```python
from build123d import *

# Parameters (mm, degrees)
AUFSATZ_LINEAR_AUSTRAGEN2_DEPTH = 5
SCHNITT_LINEAR_AUSTRAGEN2_DEPTH = 38.080992435


with BuildPart() as part:
    # Skizze1 → Aufsatz-Linear austragen2 (new body)
    with BuildSketch(Plane.XY):
        with BuildLine():
            Line((0, 0), (0, 30))
            ThreePointArc((0, 30), (11.480502971, 27.716385975), (21.213203436, 21.213203436))
            Line((21.213203436, 21.213203436), (0, 0))
        make_face()
    extrude(amount=AUFSATZ_LINEAR_AUSTRAGEN2_DEPTH)

    # Skizze2 → Schnitt-Linear austragen2 (cut, through all)
    with BuildSketch(Plane.XY.offset(5)):
        with BuildLine():
            Line((14.142135624, 14.142135624), (21.213203436, 21.213203436))
            ThreePointArc((21.213203436, 21.213203436), (15, 25.980762114), (7.764571353, 28.977774789))
            Line((7.764571353, 28.977774789), (5.176380902, 19.318516526))
            ThreePointArc((5.176380902, 19.318516526), (10, 17.320508076), (14.142135624, 14.142135624))
        make_face()
    extrude(amount=-SCHNITT_LINEAR_AUSTRAGEN2_DEPTH, mode=Mode.SUBTRACT)


solid = part.part
```
Model file for the job. Use its own axes, mm. A direction names the side the tool comes from. Coordinates: 2 decimals unless noted, no trailing zeros. Order: outer loops, then holes, each group sorted by start corner. A loop starts at its lowest first (then second) coordinate and runs counter-clockwise, first axis right, second up. Notation, with made-up numbers: M -2,26 L 12,26 A22 cw 12,42 Z; hole C 72,-27 d10. An arc over 180 degrees is marked long. Answer as CSV lines item,"result".
(1) Wall check: line 1 along X through (y, z) = (5, 3.7); line 2 along Y through (x, z) = (12.5, 1.35); line 3 along Y through (x, z) = (1.5, 3.2). Give the ranges that are in metal, low to high.
Geometry says:
line 1,"x = 0 to 5"
line 2,"y = 12.5 to 15.61"
line 3,"y = 1.5 to 29.96"
(2) Band-saw the part on A-A, the plane x = 7. List the corners of the cut face in (y, z) (3 decimals), then the cut area to 3 significant figures.
Geometry says:
outline,"M 7,0 L 18.735,0 L 18.735,5 L 7,5 Z; M 26.124,0 L 29.172,0 L 29.172,5 L 26.124,5 Z"
area,"73.9 mm2"
(3) Band-saw the part on B-B, the plane z = 3.5. List the corners of the cut face in (x, y), then the cut area to 3 significant figures.
Geometry says:
outline,"M 0,0 L 14.14,14.14 A20 ccw 5.18,19.32 L 7.76,28.98 A30 ccw 0,30 Z"
area,"223 mm2"
(4) Pull direction Y, two halves, no side cores. Call faces 1 (the cylindrical face through (9.936, 17.357, 2.535)), 2 (the flat face through (0, 15, 2)), 3 (the flat face through (7, 7, 2)): +Y half, -Y half, draft (parallel to the pull), parting line (faces both ways), or undercut.
Geometry says:
face 1,"undercut"
face 2,"draft"
face 3,"-Y half"
(5) 3-axis set-ups, long thin cutter, end or side, ignore diameter. For faces 4 (the flat face through (4, 15, 0)), 5 (the flat face through (6.49, 24.22, 2.54)): which of +Z, -Z, +X, -X, +Y, -Y reach the whole face in a straight line?
Geometry says:
face 4,"-Z, +X, -X, +Y, -Y"
face 5,"+Z, -Z, +X"
(6) Band-saw the part on C-C, the plane y = 4.5. List the corners of the cut face in (x, z), then the cut area to 3 significant figures.
Geometry says:
outline,"M 0,0 L 4.5,0 L 4.5,5 L 0,5 Z"
area,"22.5 mm2"
(7) Flat gauge pins, fed straight in: pin 1 (3 mm diameter, centred on x = 9.5, z = 3.5, fed in from -Y); pin 2 (1.5 mm diameter, centred on x = 9.5, z = 1.5, fed in from -Y); pin 3 (3 mm diameter, centred on y = 7, z = 3.5, fed in from +X). Where does each tip first touch, or does it go through?
Geometry says:
pin 1,"stops at y = 8"
pin 2,"stops at y = 8.75"
pin 3,"stops at x = 8.5"
(8) Band-saw the part on D-D, the plane x = 4.5. List the corners of the cut face in (y, z).
Geometry says:
outline,"M 4.5,0 L 29.66,0 L 29.66,5 L 4.5,5 Z"
